Check sheet for the modelled part. Datum: model origin and axes. Units: mm. Face numbers are marked on the shaded views. A direction names the side the tool comes from. Give positions to 0.01 mm unless a question says otherwise; leave off trailing zeros. Write each loop counter-clockwise with the first axis right and the second up, starting at its lowest first coordinate (ties: lowest second). Pieces come first, ordered by that corner, then holes. Notation, with made-up numbers: M 24,30.25 L 52,30.25 A19 ccw 52,49.25 Z; hole C -29.75,-37 d7. An arc over 180 degrees is marked long. Write item = value, one per line. Start each with the question number.
1) Cross-section at B-B, the plane y = 20. Record the cut outline in (x, z), plus the area to 4 significant figures.
2) Go/stop test with flat-tipped pins: pin 1 (1.5 mm diameter, centred on x = 18.5, y = 29.5, fed in from +Z); pin 2 (3.5 mm diameter, centred on y = 9, z = 34, fed in from +X); pin 3 (5 mm diameter, centred on x = 40, y = 10, fed in from +Z). Record where each tip stops, or that it passes through.
3) Cross-section at C-C, the plane z = 19.5. Record the cut outline in (x, y).
4) Cross-section at A-A, the plane z = 45. Record the cut outline in (x, y), plus the area to 3 significant figures.
5) Cross-section at D-D, the plane y = 50. Record the cut outline in (x, z), plus the area to 3 significant figures.
6) Access from +Z, -Z, +X, -X, +Y, -Y to the whole of each face (thin tool, end or side, straight path). Record for the marked faces 1 and 2.
7) Scan lines: line 1 along Z through (x, y) = (117, 31); line 2 along Y through (x, z) = (20, 1.85); line 3 along X through (y, z) = (50, 3). Record each from-to range of solid material in increasing order. Write a range as [from, to].
Solid Edge part; units mm, degrees
sketch "Sketch1" plane through (0, 0, 0) normal (0, 0, 1) x (1, 0, 0)
  line L0 (120, 60) -> (0, 60)
  line L1 (0, 60) -> (0, 0)
  line L2 (0, 0) -> (120, 0)
  line L3 (120, 0) -> (120, 60)
extrude "Protrusion1" add sketch "Sketch1" along normal blind 5
sketch "Sketch2" plane through (60, 20, 5) normal (0, 0, 1) x (1, 0, 0)
  line L0 (55, -20) -> (55, 40)
  line L1 (55, 40) -> (60, 40)
  line L2 (60, 40) -> (60, -20)
  line L3 (60, -20) -> (55, -20)
  line L4 (-55, 40) -> (-55, -20)
  line L5 (-55, -20) -> (-60, -20)
  line L6 (-60, -20) -> (-60, 40)
  line L7 (-60, 40) -> (-55, 40)
extrude "Extrusionsausprägung_2" add sketch "Sketch2" along normal blind 60
hole "Bohrung_1" at (120, 20, 45) direction (-1, 0, 0) diameter 19 end up to next
hole "Hole_2" at (20, 10, 5) direction (0, 0, -1) diameter 4.2 end up to next start chamfer 0.6 start chamfer angle 45
hole "Hole1" at (20, 50, 5) direction (0, 0, -1) diameter 4.2 end up to next start chamfer 0.6 start chamfer angle 45
hole "Hole2" at (40, 50, 5) direction (0, 0, -1) diameter 4.2 end up to next start chamfer 0.6 start chamfer angle 45
hole "Hole3" at (40, 10, 5) direction (0, 0, -1) diameter 4.2 end up to next start chamfer 0.6 start chamfer angle 45
hole "Hole4" at (120, 9, 56) direction (-1, 0, 0) diameter 4.2 end up to next
hole "Hole5" at (120, 9, 34) direction (-1, 0, 0) diameter 4.2 end up to next
hole "Hole6" at (120, 31, 34) direction (-1, 0, 0) diameter 4.2 end up to next
hole "Hole7" at (120, 31, 56) direction (-1, 0, 0) diameter 4.2 end up to next
hole "Hole_10" at (0, 20, 45) direction (1, 0, 0) diameter 16 end up to next
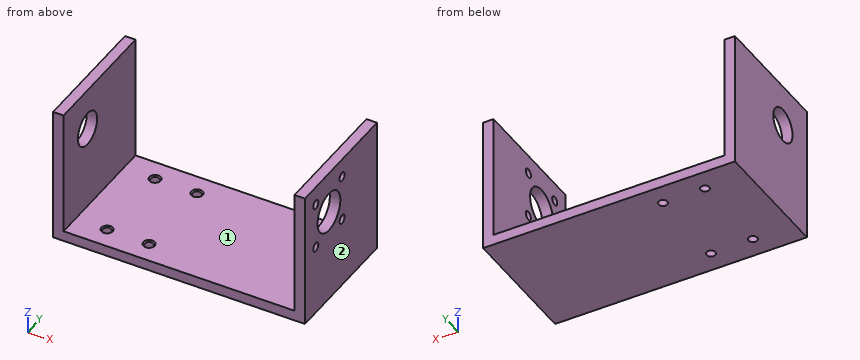
Reply:
q1.outline = M 0,0 L 120,0 L 120,35.5 L 115,35.5 L 115,5 L 5,5 L 5,37 L 0,37 Z; M 0,53 L 5,53 L 5,65 L 0,65 Z; M 115,54.5 L 120,54.5 L 120,65 L 115,65 Z
q1.area = 1,025 mm2
q2.pin_1 = 5
q2.pin_2 = 5
q2.pin_3 = 4.8
q3.outline = M 0,0 L 5,0 L 5,60 L 0,60 Z; M 115,0 L 120,0 L 120,60 L 115,60 Z
q4.outline = M 0,0 L 5,0 L 5,12 L 0,12 Z; M 0,28 L 5,28 L 5,60 L 0,60 Z; M 115,0 L 120,0 L 120,10.5 L 115,10.5 Z; M 115,29.5 L 120,29.5 L 120,60 L 115,60 Z
q4.area = 425 mm2
q5.outline = M 0,0 L 17.9,0 L 17.9,4.4 L 17.3,5 L 5,5 L 5,65 L 0,65 Z; M 22.1,0 L 37.9,0 L 37.9,4.4 L 37.3,5 L 22.7,5 L 22.1,4.4 Z; M 42.1,0 L 120,0 L 120,65 L 115,65 L 115,5 L 42.7,5 L 42.1,4.4 Z
q5.area = 1,160 mm2
q6.face_1 = +Z, +Y, -Y
q6.face_2 = +Z, -Z, +X, +Y, -Y
q7.line_1 = [0, 31.9], [36.1, 53.9], [58.1, 65]
q7.line_2 = [0, 7.9], [12.1, 47.9], [52.1, 60]
q7.line_3 = [0, 17.9], [22.1, 37.9], [42.1, 120]
